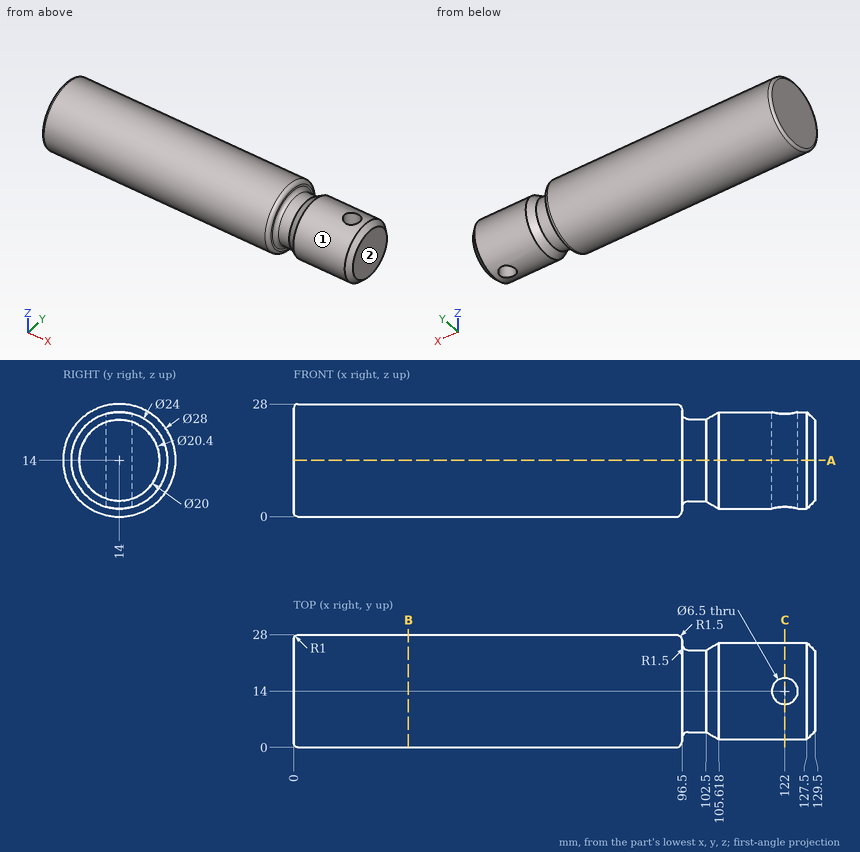
For this review, use the dimensioned drawing (mm, ordinates from the lowest corner) and the shaded views. A direction names the side the tool comes from. Give positions to 0.01 mm unless a question says otherwise; leave off trailing zeros. Write each loop counter-clockwise with the first axis right and the second up, starting at its lowest first coordinate (ties: lowest second). Pieces come first, ordered by that corner, then holes. Notation, with made-up numbers: M -31.5,83.25 L -12.5,83.25 A20 cw -12.5,110.25 Z; hole C 61,73.5 d6. An arc over 180 degrees is marked long. Answer as a JSON object with one key per item and string values. Group by question number.
Item 1: For probe 1 along Z at (x, y) = (85, 14.75); probe 2 along Z at (x, y) = (69, 7.75); probe 3 along X at (y, z) = (11.25, 17.25), list the stretches that pass through material, from the lowest coordinate up. Write a range as [from, to].
Item 2: For pin 1 Ø3 at (x, z) = (52.5, 6) entering from -Y; pin 2 Ø12 at (x, y) = (110, 12.5) entering from -Z; pin 3 Ø1.5 at (x, z) = (60.5, 8) entering from +Y, all flat-tipped, find the tip position at first contact; note any pin that passes through.
Item 3: Tool access review of the marked faces 1 and 2: name each direction out of +Z, -Z, +X, -X, +Y, -Y from which nothing blocks a thin tool from reaching the whole face with its end or side.
Item 4: Consider section A-A on z = 14. Write out the cut boundary in (x, y), plus the area to 3 significant figures.
Item 5: Consider section C-C on x = 122. Write out the cut boundary in (y, z).
Item 6: Consider section B-B on x = 28.5. Write out the cut boundary in (y, z), plus the area to 3 significant figures.
Check result:
{
 "1": {"probe 1": "z = [0.02, 27.98]", "probe 2": "z = [1.47, 26.53]", "probe 3": "x = [0, 120.27], [123.73, 129.5]"},
 "2": {"pin 1": "stops at y = 1.6", "pin 2": "stops at z = 2", "pin 3": "stops at y = 26.98"},
 "3": {"face 1": "+X", "face 2": "+Z, -Z, +X, +Y, -Y"},
 "4": {"outline": "M 0,1 A1 ccw 1,0 L 95,0 A1.5 ccw 96.5,1.5 L 96.5,2.3 A1.5 cw 98,3.8 L 102.5,3.8 L 105.62,2 L 127.5,2 L 129.5,4 L 129.5,24 L 127.5,26 L 105.62,26 L 102.5,24.2 L 98,24.2 A1.5 cw 96.5,25.7 L 96.5,26.5 A1.5 ccw 95,28 L 1,28 A1 ccw 0,27 Z; hole C 122,14 d6.5", "area": "3,430 mm^2"},
 "5": {"outline": "M 10.75,2.45 L 10.75,25.55 A12 ccw Z; M 17.25,2.45 A12 ccw 17.25,25.55 Z"},
 "6": {"outline": "C 14,14 d28", "area": "616 mm^2"}
}
